Check sheet for the modelled part. Datum: model origin and axes. Units: mm. Face numbers are marked on the shaded views. Round coordinates to 2 decimals unless told otherwise and drop trailing zeros. Order: outer loops, then holes, each group sorted by start corner. A loop starts at its lowest first (then second) coordinate and runs counter-clockwise, first axis right, second up. Notation, with made-up numbers: (-24, 9.5) -> (14, 9.5) arc R9 ccw to (14, 19.5) -> close; hole circle Ø11 at (0.25, 31.25). An arc over 180 degrees is marked (long way). Answer in a Markdown table with one row per item. Add a question column.
1. Draft check along X on the marked faces 1, 2 and 3. Enter one of: +X half, -X half, draft (parallel to the pull), parting line (faces both ways), or undercut.
2. Sectioned sample at A-A, the plane y = 0. Record the boundary of the cut face in (x, z).
3. Sectioned sample at D-D, the plane z = -18. Record the boundary of the cut face in (x, y) (1 decimal).
4. Material ranges on L1, parallel to Y at x = 0, z = 11; L2, parallel to Z at x = 2.5, y = 1; L3, parallel to Y at x = 1.5, z = -7, recorded low to high. Write a range as from..to.
5. Sectioned sample at C-C, the plane z = -5. Record the boundary of the cut face in (x, y) (1 decimal).
6. Depth check by flat-ended pin: P1, Ø1, axis at x = -4, z = -6, coming from the +Y side; P2, Ø1.5, axis at y = -2, z = 1, coming from the +X side; P3, Ø6.5, axis at x = 0.5, y = 0.5, coming from the +Z side; P4, Ø8, axis at y = 6, z = -12, coming from the +X side. Enter the tip coordinate at first touch or a pass-through.
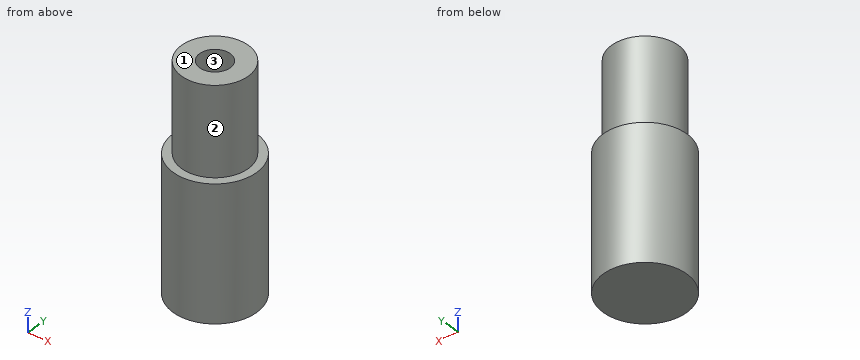
Autodesk Inventor part; units mm, degrees
ref_plane "YZ Plane" through (0, 0, 0) normal (1, 0, 0) x (0, 1, 0)
ref_plane "XZ Plane" through (0, 0, 0) normal (0, 1, 0) x (-1, 0, 0)
ref_plane "XY Plane" through (0, 0, 0) normal (0, 0, 1) x (1, 0, 0)
sketch "Sketch1" plane through (0, 0, 0) normal (0, 0, 1) x (1, 0, 0)
  circle A0 centre (0, 0) radius 7.9375
  circle A1 centre (0, 0) radius 6.35
  dimension "d0" = 15.875
  dimension "d1" = 12.7
extrude "Extrusion1" add sketch "Sketch1" against normal blind 25.4 contours A0 | A1
extrude "Extrusion2" add sketch "Sketch1" along normal blind 16.764 contours A1
thread "Thread1"
sketch "Sketch2" plane through (0, 0, 16.764) normal (0, 0, 1) x (1, 0, 0)
  circle A0 centre (0, 0) radius 6.35
  circle A1 centre (0, 0) radius 2.921
  dimension "d8" = 5.842
extrude "Extrusion3" cut sketch "Sketch2" against normal blind 25.4 contours A1
thread "Thread2"
properties part number "PDewalt Drill Shaft .5in"
Answer key:
| question | item | result |
|---|---|---|
| 1 | face 1 | draft |
| 1 | face 2 | parting line |
| 1 | face 3 | undercut |
| 2 | outline | (-7.94, -25.4) -> (7.94, -25.4) -> (7.94, 0) -> (6.35, 0) -> (6.35, 16.76) -> (2.92, 16.76) -> (2.92, -8.64) -> (-2.92, -8.64) -> (-2.92, 16.76) -> (-6.35, 16.76) -> (-6.35, 0) -> (-7.94, 0) -> close |
| 3 | outline | circle Ø15.9 at (0, 0) |
| 4 | L1 | y = -6.35..-2.92, 2.92..6.35 |
| 4 | L2 | z = -25.4..-8.64 |
| 4 | L3 | y = -7.79..-2.51, 2.51..7.79 |
| 5 | outline | circle Ø15.9 at (0, 0); hole circle Ø5.8 at (0, 0) |
| 6 | P1 | stops at y = 7.12 |
| 6 | P2 | stops at x = 6.23 |
| 6 | P3 | stops at z = 16.76 |
| 6 | P4 | stops at x = 7.68 |
